Autodesk Inventor part; units mm, degrees
ref_plane "YZ Plane" through (0, 0, 0) normal (1, 0, 0) x (0, 1, 0)
ref_plane "XZ Plane" through (0, 0, 0) normal (0, 1, 0) x (-1, 0, 0)
ref_plane "XY Plane" through (0, 0, 0) normal (0, 0, 1) x (1, 0, 0)
sketch "Sketch1" plane through (0, 0, 0) normal (0, 0, 1) x (1, 0, 0)
  circle A0 centre (0, 0) radius 8.0328
  circle A1 centre (0, 0) radius 10.5727
  dimension "d0" = 16.0655
  dimension "d3" = 2.54
extrude "Extrusion1" add sketch "Sketch1" along normal blind 6.35
sketch "Sketch3" plane through (0, 0, 6.35) normal (0, 0, 1) x (1, 0, 0)
  circle A0 centre (0, 0) radius 10.5727
  circle A1 centre (0, 0) radius 10.5727
  circle A2 centre (0, 0) radius 8.0328
  circle A3 centre (0, 0) radius 8.0328
extrude "Extrusion2" add sketch "Sketch3" along normal blind 6.2738
sketch "Sketch7" plane through (0, 0, 12.6238) normal (0, 0, 1) x (1, 0, 0)
  circle A0 centre (0, 0) radius 10.5727
  circle A1 centre (0, 0) radius 7.5882
  dimension "d12" = 15.1765
extrude "Extrusion4" add sketch "Sketch7" along normal blind 6.858
sketch "Sketch8" plane through (0, 0, 19.4818) normal (0, 0, 1) x (1, 0, 0)
  circle A0 centre (0, 0) radius 10.5727
  circle A1 centre (0, 0) radius 5.0864
  dimension "d15" = 10.1727
extrude "Extrusion5" add sketch "Sketch8" along normal blind 3.5179
properties part number "Magnet to Igus adapter"
Design review of the part built by this model. Coordinates are the model's own, in mm. A direction names the side the tool comes from. Round coordinates to 2 decimals unless told otherwise and drop trailing zeros. Write each loop counter-clockwise with the first axis right and the second up, starting at its lowest first coordinate (ties: lowest second). Pieces come first, ordered by that corner, then holes. Notation, with made-up numbers: (16.5, 40.5) - (41.5, 40.5) arc R14 cw to (41.5, 64.5) - close; hole circle Ø2 at (-28.75, 10). An arc over 180 degrees is marked (long way). Use a Markdown table: item, result. Add a question column.
1. Mouldability with a two-part tool opening along Y and no side actions: class faces 3 (the face through (-7.79, -7.15, 11.34)), 4 (the face through (-2, 8, 0)), 5 (the face through (5, -2, 19.482)) as +Y half, -Y half, draft (parallel to the pull), parting line (faces both ways), or undercut.
2. Wall thickness on probe 1 along Y at (x, z) = (0, 15.75); probe 2 along Y at (x, z) = (0, 4.5); probe 3 along X at (y, z) = (4.5, 20.5): over which ranges is each line inside the solid? List them lowest first.
3. We need section A-A (x = 0). State the section outline as (y, z) points, then the cut area to 3 significant figures.
4. For faces 1 (the face through (-1.741, 7.842, 6.224)), 2 (the face through (5, 2, 23)), list the 3-axis set-ups (+Z, -Z, +X, -X, +Y, -Y) from which the entire face can be reached by the end or side of a thin tool; tool diameter is ignored.
5. We need section C-C (z = 20). State the section outline as (x, y) points, then the cut area to 3 significant figures.
6. Clearance check with flat-ended pins moving along their axes: pin 1 (5 mm diameter, centred on x = 3, y = 0, fed in from -Z); pin 2 (8 mm diameter, centred on x = 0, y = 0, fed in from -Z); pin 3 (8 mm diameter, centred on x = -4.5, z = 9, fed in from -Y); pin 4 (1 mm diameter, centred on y = 2, z = 5, fed in from +X). State where each tip first meets the part, or that it passes through.
7. We need section D-D (z = 16). State the section outline as (x, y) points.
Output:
| question | item | result |
|---|---|---|
| 1 | face 3 | parting line |
| 1 | face 4 | draft |
| 1 | face 5 | undercut |
| 2 | probe 1 | y = -10.57 to -7.59, 7.59 to 10.57 |
| 2 | probe 2 | y = -10.57 to -8.03, 8.03 to 10.57 |
| 2 | probe 3 | x = -9.57 to -2.37, 2.37 to 9.57 |
| 3 | outline | (-10.57, 0) - (-8.03, 0) - (-8.03, 12.62) - (-7.59, 12.62) - (-7.59, 19.48) - (-5.09, 19.48) - (-5.09, 23) - (-10.57, 23) - close; (5.09, 19.48) - (7.59, 19.48) - (7.59, 12.62) - (8.03, 12.62) - (8.03, 0) - (10.57, 0) - (10.57, 23) - (5.09, 23) - close |
| 3 | area | 144 mm2 |
| 4 | face 1 | -Z |
| 4 | face 2 | +Z, +X, -X, +Y, -Y |
| 5 | outline | circle Ø21.15 at (0, 0); hole circle Ø10.17 at (0, 0) |
| 5 | area | 270 mm2 |
| 6 | pin 1 | stops at z = 19.48 |
| 6 | pin 2 | passes through |
| 6 | pin 3 | stops at y = -10.56 |
| 6 | pin 4 | stops at x = 10.47 |
| 7 | outline | circle Ø21.15 at (0, 0); hole circle Ø15.18 at (0, 0) |
